Here's how the part is built. I have some questions about the finished solid (model axes, mm). Face numbers are marked on the shaded views. A direction names the side the tool comes from. Coordinates: 2 decimals unless noted, no trailing zeros. Write each loop counter-clockwise with the first axis right and the second up, starting at its lowest first coordinate (ties: lowest second). Pieces come first, ordered by that corner, then holes. Notation, with made-up numbers: (-37, 22) -> (-28, 22) arc R18 ccw to (-28, 37) -> close; hole circle Ø2 at (14, 36.25). An arc over 180 degrees is marked (long way). Put each result on its own line as item: value. Start each with the question number.
Item 1: I need wall thicknesses on line 1 (Z direction, x = 0, y = -18); line 2 (Y direction, x = -4.5, z = -26); line 3 (Y direction, x = 0, z = 6.25). Which ranges of each line are inside material? Lowest first, please. Write a range as [from, to].
Item 2: If we mould it in two halves opening along X, with no side actions, what happens to the marked faces 1, 2, 3 and 4? For each: released by +X, released by -X, zero draft, split by the parting line, or undercut.
Item 3: I want a section at D-D, the plane x = -16. List the corners of the cut face in (y, z) for me.
Item 4: I want a section at B-B, the plane x = 0. List the corners of the cut face in (y, z) for me, then the cut area to 3 significant figures.
Item 5: On a 3-axis mill with a long thin cutter (end or side, diameter ignored), from which of +Z, -Z, +X, -X, +Y, -Y can I reach the whole of each face in a straight line? I mean the marked faces 5, 6, 7 and 8. Say none if no direction works.
Item 6: For pin 1 (1.6 mm diameter, centred on y = -20.5, z = -23, fed in from +X); pin 2 (3.5 mm diameter, centred on x = -2, z = -23, fed in from -Y); pin 3 (1.6 mm diameter, centred on y = -22, z = -23, fed in from -X), each with a flat end and sliding along its axis, tell me the tip position at first contact or that it passes through.
Item 7: I want a section at C-C, the plane z = -30.35. List the corners of the cut face in (x, y) for me, then the cut area to 3 significant figures.
Item 8: I want a section at A-A, the plane y = 0. List the corners of the cut face in (x, z) for me.
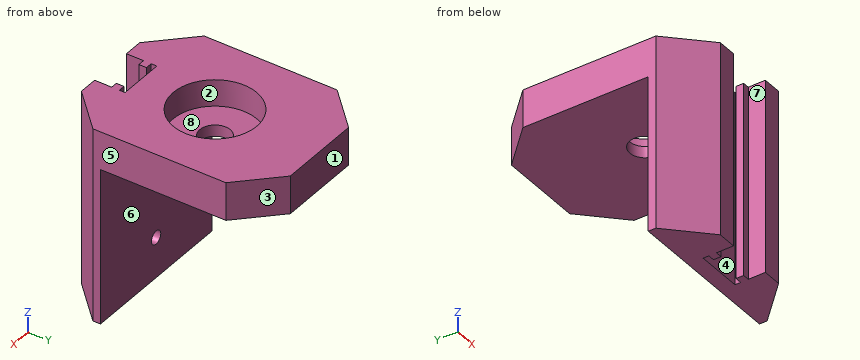
from build123d import *

# Parameters (mm, degrees)
ESTRUSIONE_ESTRUSIONE1_DEPTH = 10
SCHIZZO2_R                   = 11
TAGLIO_ESTRUSIONE1_DEPTH     = 7
SCHIZZO3_R                   = 4
TAGLIO_ESTRUSIONE2_DEPTH     = 4
ESTRUSIONE_ESTRUSIONE2_DEPTH = 41
SMUSSO1_SIZE                 = 10
SCHIZZO5_R                   = 1.75
TAGLIO_ESTRUSIONE3_DEPTH     = 13


with BuildPart() as part:
    # Schizzo1 → Estrusione-Estrusione1 (new body)
    with BuildSketch(Plane.XY):
        Polygon((6, -23), (6, -27.5), (21, -27.5), (21, 27.5), (-21, 27.5), (-21, -27.5), (-6, -27.5), (-6, -23), (-4.25, -23), (-4.25, -21), (-6, -21), (-6, -19.5), (6, -19.5), (6, -21), (4.25, -21), (4.25, -23), align=None)
    extrude(amount=ESTRUSIONE_ESTRUSIONE1_DEPTH)

    # Schizzo2 → Taglio-Estrusione1 (cut)
    with BuildSketch(Plane.XY.offset(10)):
        Circle(SCHIZZO2_R)
    extrude(amount=-TAGLIO_ESTRUSIONE1_DEPTH, mode=Mode.SUBTRACT)

    # Schizzo3 → Taglio-Estrusione2 (cut, through all)
    with BuildSketch(Plane.XY.offset(3)):
        Circle(SCHIZZO3_R)
    extrude(amount=-TAGLIO_ESTRUSIONE2_DEPTH, mode=Mode.SUBTRACT)

    # Schizzo4 → Estrusione-Estrusione2 (add)
    with BuildSketch(Plane(origin=(0, 0, 0), x_dir=(-1, 0, 0), z_dir=(0, 0, -1))):
        Polygon((-21, -27.5), (-6, -27.5), (-6, -23), (-4.25, -23), (-4.25, -21), (-6, -21), (-6, -19.5), (6, -19.5), (6, -21), (4.25, -21), (4.25, -23), (6, -23), (6, -27.5), (21, -27.5), (21, -15.5), (-21, -15.5), align=None)
    extrude(amount=ESTRUSIONE_ESTRUSIONE2_DEPTH)

    # Smusso1
    smusso1_edges = [part.edges().sort_by_distance(p)[0] for p in [
        (21, -27.5, -15.5),
        (-21, -27.5, -15.5),
        (-21, 27.5, 5),
        (21, 27.5, 5),
    ]]
    chamfer(smusso1_edges, length=SMUSSO1_SIZE)

    # Schizzo5 → Taglio-Estrusione3 (cut, through all)
    with BuildSketch(Plane(origin=(0, -15.5, 0), x_dir=(1, 0, 0), z_dir=(0, 1, 0))):
        with Locations((0, 30.35)):
            Circle(SCHIZZO5_R)
        with Locations((0, 5.35)):
            Circle(SCHIZZO5_R)
    extrude(amount=-TAGLIO_ESTRUSIONE3_DEPTH, mode=Mode.SUBTRACT)


solid = part.part
Calculated:
1. line 1: z = [-41, -32.1], [-28.6, -7.1], [-3.6, 10]
1. line 2: y = [-23, -21], [-19.5, -15.5]
1. line 3: y = [-19.5, -11], [11, 27.5]
2. face 1: zero draft
2. face 2: undercut
2. face 3: released by +X
2. face 4: undercut
3. outline: (-22.5, -41) -> (-15.5, -41) -> (-15.5, 0) -> (22.5, 0) -> (22.5, 10) -> (-22.5, 10) -> close
4. outline: (-19.5, -41) -> (-15.5, -41) -> (-15.5, -32.1) -> (-19.5, -32.1) -> close; (-19.5, -28.6) -> (-15.5, -28.6) -> (-15.5, -7.1) -> (-19.5, -7.1) -> close; (-19.5, -3.6) -> (-15.5, -3.6) -> (-15.5, 0) -> (-4, 0) -> (-4, 3) -> (-11, 3) -> (-11, 10) -> (-19.5, 10) -> close; (4, 0) -> (27.5, 0) -> (27.5, 10) -> (11, 10) -> (11, 3) -> (4, 3) -> close
4. area: 428 mm2
5. face 5: +Z, -Z, +X, +Y, -Y
5. face 6: -Z, +X, -X, +Y
5. face 7: +Z, -Z, -Y
5. face 8: +Z
6. pin 1: stops at x = 18.8
6. pin 2: stops at y = -19.5
6. pin 3: stops at x = -17.3
7. outline: (-21, -17.5) -> (-11, -27.5) -> (-6, -27.5) -> (-6, -23) -> (-4.25, -23) -> (-4.25, -21) -> (-6, -21) -> (-6, -19.5) -> (-1.75, -19.5) -> (-1.75, -15.5) -> (-21, -15.5) -> close; (1.75, -19.5) -> (6, -19.5) -> (6, -21) -> (4.25, -21) -> (4.25, -23) -> (6, -23) -> (6, -27.5) -> (11, -27.5) -> (21, -17.5) -> (21, -15.5) -> (1.75, -15.5) -> close
7. area: 301 mm2
8. outline: (-21, 0) -> (-4, 0) -> (-4, 3) -> (-11, 3) -> (-11, 10) -> (-21, 10) -> close; (4, 0) -> (21, 0) -> (21, 10) -> (11, 10) -> (11, 3) -> (4, 3) -> close
